Here's how the part is built. I have some questions about the finished solid (model axes, mm). Give positions to 0.01 mm unless a question says otherwise; leave off trailing zeros. Order: outer loops, then holes, each group sorted by start corner. A loop starts at its lowest first (then second) coordinate and runs counter-clockwise, first axis right, second up. Notation, with made-up numbers: M -17,58.5 L -6,58.5 A15 cw -6,86.5 Z; hole C -12.5,27 d4. An arc over 180 degrees is marked long. Use one line per item in the form item = value.
Autodesk Inventor part; units mm, degrees
ref_plane "YZ Plane" through (0, 0, 0) normal (1, 0, 0) x (0, 1, 0)
ref_plane "XZ Plane" through (0, 0, 0) normal (0, 1, 0) x (-1, 0, 0)
ref_plane "XY Plane" through (0, 0, 0) normal (0, 0, 1) x (1, 0, 0)
sketch "Sketch1" plane through (0, 0, 0) normal (0, 1, 0) x (-1, 0, 0)
  line L0 (-8, -3) -> (8, -3)
  line L1 (8, -3) -> (8, 3)
  line L2 (8, 3) -> (-8, 3)
  line L3 (-8, 3) -> (-8, -3)
  line L4 (-8, -3) -> (8, 3) construction
  line L5 (8, -3) -> (-8, 3) construction
  circle A0 centre (8, 0) radius 3
  circle A1 centre (-8, 0) radius 3
  point P0 (0, 0)
  dimension "d0" = 16
  dimension "d1" = 6
  dimension "d2" = 6
  dimension "d3" = 6
extrude "Extrusion1" add sketch "Sketch1" along normal blind 2
sketch "Sketch2" plane through (0, 2, 0) normal (0, 1, 0) x (1, 0, 0)
  arc A0 (8, -3) -> (8, 3) centre (8, 0) ccw
  arc A1 (-8, 3) -> (-8, -3) centre (-8, 0) ccw
  circle A2 centre (-8, 0) radius 1.5
  circle A3 centre (8, 0) radius 1.5
  point P0 (0, 0)
  dimension "d6" = 3
  dimension "d7" = 3
extrude "Extrusion2" cut sketch "Sketch2" against normal blind 2
sketch "Sketch3" plane through (0, 0, 0) normal (0, -1, 0) x (1, 0, 0)
  circle A0 centre (-8, 0) radius 1.5
  circle A1 centre (8, 0) radius 1.5
  arc A2 (8, -3) -> (8, 3) centre (8, 0) ccw
  arc A3 (-8, 3) -> (-8, -3) centre (-8, 0) ccw
  circle A4 centre (-8, 0) radius 0.1
  circle A5 centre (8, 0) radius 0.1
  point P0 (0, 0)
  dimension "d10" = 0.2
  dimension "d11" = 0.2
extrude "Extrusion3" add sketch "Sketch3" against normal blind 2
properties part number "tahlo5(b)_sablona"
Q1. I want a section at B-B on z = -2. Write out the boundary of the cut face in (x, y).
Found:
outline = M -10.24,0 L 10.24,0 L 10.24,2 L -10.24,2 Z
Q2. I want a section at C-C on z = 1.95. Write out the boundary of the cut face in (x, y).
Found:
outline = M -10.28,0 L 10.28,0 L 10.28,2 L -10.28,2 Z
Q3. I want a section at A-A on y = 1.6. Write out the boundary of the cut face in (x, z), then the cut area to 3 significant figures.
Found:
outline = M -8,-3 L 8,-3 A3 ccw 8,3 L -8,3 A3 ccw Z; hole C -8,0 d0.2; hole C 8,0 d0.2
area = 124 mm²
Q4. I need wall thicknesses on L1, parallel to Z at x = 8, y = 0.8; L2, parallel to X at y = 1.8, z = -0.05; L3, parallel to X at y = 1.7, z = 0.7. Which ranges of each line are inside material? Lowest first, please.
Found:
L1 = -3 to -0.1, 0.1 to 3
L2 = -11 to -8.09, -7.91 to 7.91, 8.09 to 11
L3 = -10.92 to 10.92
